Part model, mm, in its own coordinate system. Round coordinates to 2 decimals unless told otherwise and drop trailing zeros. Loops run counter-clockwise (first coordinate to the right, second up) from the corner with the lowest first, then second, coordinate; pieces in that order, holes last. Notation, with made-up numbers: (45.5, 44) -> (49.5, 44) arc R29 ccw to (49.5, 72) -> close; hole circle Ø9 at (83.25, -19.75). An arc over 180 degrees is marked (long way). Answer as CSV lines item,"result".
from build123d import *

# Parameters (mm, degrees)
SKETCH1_W               = 125
SKETCH1_H               = 75
SKETCH1_W_2             = 22
SKETCH1_H_2             = 22
BOSS_EXTRUDE1_DEPTH     = 1.2
SKETCH2_W               = 3
SKETCH2_H               = 22
CUT_EXTRUDE1_DEPTH      = 1
CUT_EXTRUDE1_DEPTH_BACK = 2.2


with BuildPart() as part:
    # Sketch1 → Boss-Extrude1 (new body)
    with BuildSketch(Plane(origin=(0, 0, 0), x_dir=(1, 0, 0), z_dir=(0, 1, 0))):
        Rectangle(SKETCH1_W, SKETCH1_H)
        with Locations((14.8, -8)):
            Rectangle(SKETCH1_W_2, SKETCH1_H_2, mode=Mode.SUBTRACT)
    extrude(amount=BOSS_EXTRUDE1_DEPTH)

    # Sketch2 → Cut-Extrude1 (cut, two sides)
    with BuildSketch(Plane(origin=(0, 1.2, 0), x_dir=(1, 0, 0), z_dir=(0, 1, 0))) as cut_extrude1_sk:
        with Locations((27.3, -8)):
            Rectangle(SKETCH2_W, SKETCH2_H)
    extrude(amount=CUT_EXTRUDE1_DEPTH, mode=Mode.SUBTRACT)
    extrude(cut_extrude1_sk.sketch, amount=-CUT_EXTRUDE1_DEPTH_BACK, mode=Mode.SUBTRACT)


solid = part.part
Q1. Drill centre lines: line 1 along Z through (x, y) = (27, 0.75); line 2 along X through (y, z) = (0.95, 13.5). Where is each one in solid material? Low to high.
Geometry results:
line 1,"-37.5 to -3, 19 to 37.5"
line 2,"-62.5 to 3.8, 28.8 to 62.5"
Q2. Saw through at B-B, the plane y = 0.45. Write the cut outline in (x, z), then the cut area to 4 significant figures.
Geometry results:
outline,"(-62.5, -37.5) -> (62.5, -37.5) -> (62.5, 37.5) -> (-62.5, 37.5) -> close; hole (3.8, -3) -> (28.8, -3) -> (28.8, 19) -> (3.8, 19) -> close"
area,"8,825 mm2"
Q3. Saw through at C-C, the plane z = 10.5. Write the cut outline in (x, y).
Geometry results:
outline,"(-62.5, 0) -> (3.8, 0) -> (3.8, 1.2) -> (-62.5, 1.2) -> close; (28.8, 0) -> (62.5, 0) -> (62.5, 1.2) -> (28.8, 1.2) -> close"
Q4. Saw through at A-A, the plane x = 7.5. Write the cut outline in (y, z).
Geometry results:
outline,"(0, -37.5) -> (1.2, -37.5) -> (1.2, -3) -> (0, -3) -> close; (0, 19) -> (1.2, 19) -> (1.2, 37.5) -> (0, 37.5) -> close"
